from build123d import *

# Parameters (mm, degrees)
F1_DEPTH = 9
F0_R     = 2.5
F2_DEPTH = 2
F3_DEPTH = 6
F4_START = 6
F0_R_2   = 2
F4_DEPTH = 3
F5_W     = 2
F5_H     = 3
F6_DEPTH = 6


with BuildPart() as f1:
    # F0 (on Top) → F1 (new body)
    with BuildSketch(Plane.XY):
        Polygon((-4.9984134711, 16), (-23.5, 16), (-23.5, -16), (-4.9984134711, -16), (4.9998776676, -16), (23.5, -16), (23.5, 16), (4.9998776676, 16), align=None)
        Polygon((-21.5, 11), (-21.5, 14), (-18.5, 14), (18.5, 14), (21.5, 14), (21.5, 11), (21.5, -11), (21.5, -14), (18.5, -14), (-18.5, -14), (-21.5, -14), (-21.5, -11), align=None, mode=Mode.SUBTRACT)
    extrude(amount=F1_DEPTH)

    # F0 (on Top) → F2 (join)
    with BuildSketch(Plane.XY):
        with BuildLine():
            Line((18.5, 14), (-18.5, 14))
            ThreePointArc((-18.5, 14), (-19.3786796564, 11.8786796564), (-21.5, 11))
            Line((-21.5, 11), (-21.5, -11))
            ThreePointArc((-21.5, -11), (-19.3786796564, -11.8786796564), (-18.5, -14))
            Line((-18.5, -14), (18.5, -14))
            ThreePointArc((18.5, -14), (19.3786796564, -11.8786796564), (21.5, -11))
            Line((21.5, -11), (21.5, 11))
            ThreePointArc((21.5, 11), (19.3786796564, 11.8786796564), (18.5, 14))
        make_face()
        with Locations((-11.5, 0)):
            Circle(F0_R, mode=Mode.SUBTRACT)
    extrude(amount=F2_DEPTH)

    # F0 (on Top) → F3 (join)
    with BuildSketch(Plane.XY):
        with BuildLine():
            Line((-18.5, 14), (-21.5, 14))
            Line((-21.5, 14), (-21.5, 11))
            ThreePointArc((-21.5, 11), (-19.3786796564, 11.8786796564), (-18.5, 14))
        make_face()
        with BuildLine():
            Line((21.5, 14), (18.5, 14))
            ThreePointArc((18.5, 14), (19.3786796564, 11.8786796564), (21.5, 11))
            Line((21.5, 11), (21.5, 14))
        make_face()
        with BuildLine():
            Line((21.5, -14), (21.5, -11))
            ThreePointArc((21.5, -11), (19.3786796564, -11.8786796564), (18.5, -14))
            Line((18.5, -14), (21.5, -14))
        make_face()
        with BuildLine():
            ThreePointArc((-18.5, -14), (-19.3786796564, -11.8786796564), (-21.5, -11))
            Line((-21.5, -11), (-21.5, -14))
            Line((-21.5, -14), (-18.5, -14))
        make_face()
    extrude(amount=F3_DEPTH)

    # F0 (on Top) → F4 (join)
    with BuildSketch(Plane.XY.offset(F4_START)):
        with BuildLine():
            Line((-4.9984134711, 20.8740525043), (-4.9984134711, 16))
            Line((-4.9984134711, 16), (4.9998776676, 16))
            Line((4.9998776676, 16), (4.9998776676, 20.9650241638))
            ThreePointArc((4.9998776676, 20.9650241638), (5, 21), (4.9998776676, 21.0349758362))
            ThreePointArc((4.9998776676, 21.0349758362), (-0.0804649964, 25.9993524965), (-4.9984134711, 20.8740525043))
        make_face()
        with Locations((0, 21)):
            Circle(F0_R_2, mode=Mode.SUBTRACT)
        with BuildLine():
            Line((4.9998776676, -16), (-4.9984134711, -16))
            Line((-4.9984134711, -16), (-4.9984134711, -20.8740525043))
            ThreePointArc((-4.9984134711, -20.8740525043), (-0.0804649964, -25.9993524965), (4.9998776676, -21.0349758362))
            Line((4.9998776676, -21.0349758362), (4.9998776676, -20.9650241638))
            Line((4.9998776676, -20.9650241638), (4.9998776676, -16))
        make_face()
        with Locations((0, -21)):
            Circle(F0_R_2, mode=Mode.SUBTRACT)
    extrude(amount=F4_DEPTH)

    # F5 (on face) → F6 (cut)
    with BuildSketch(Plane.XY.offset(9)):
        with Locations((-22.5, 0)):
            Rectangle(F5_W, F5_H)
        with Locations((22.5, 0)):
            Rectangle(F5_W, F5_H)
    extrude(amount=-F6_DEPTH, mode=Mode.SUBTRACT)


solid = f1.part
Read the model definition and answer for the solid it produces. Units are mm, in the model's axes. A direction names the side the tool comes from. Round coordinates to 2 decimals unless told otherwise and drop trailing zeros. Write each loop counter-clockwise with the first axis right and the second up, starting at its lowest first coordinate (ties: lowest second). Pieces come first, ordered by that corner, then holes.
Q1. Find section C-C on z = 0.75. Determine the outline of the cut face in (x, y), and give its area (3 significant figures).
Values:
outline: (-23.5, -16) - (23.5, -16) - (23.5, 16) - (-23.5, 16) - close; hole circle Ø5 at (-11.5, 0)
area: 1,480 mm2
Q2. Find section A-A on y = 0. Determine the outline of the cut face in (x, z).
Values:
outline: (-23.5, 0) - (-14, 0) - (-14, 2) - (-21.5, 2) - (-21.5, 3) - (-23.5, 3) - close; (-9, 0) - (23.5, 0) - (23.5, 3) - (21.5, 3) - (21.5, 2) - (-9, 2) - close
Q3. The mould has two halves that part along X. Classify faces 1 (the face through (-19.4, 11.86, 3.97)), 2 (the face through (0, 0, 0)), 3 (the face through (-23.5, 0, 2)): released by +X, released by -X, zero draft, split by the parting line, or undercut.
Values:
face 1: undercut
face 2: zero draft
face 3: released by -X
Q4. Find section B-B on x = -11.5. Determine the outline of the cut face in (y, z).
Values:
outline: (-16, 0) - (-2.5, 0) - (-2.5, 2) - (-14, 2) - (-14, 9) - (-16, 9) - close; (2.5, 0) - (16, 0) - (16, 9) - (14, 9) - (14, 2) - (2.5, 2) - close
Q5. A tool of negligible diameter and unlimited length cuts with its end or side. For faces 4 (the face through (-0.1, -18.7, 6)), 5 (the face through (-23, 0, 3)), 6 (the face through (20, 13, 6)), 7 (the face through (-4.998, 18, 7)), from which of +Z, -Z, +X, -X, +Y, -Y can it reach the whole face along a straight path? Write none if from no direction.
Values:
face 4: -Z, +X, -X, -Y
face 5: +Z, +X, -X
face 6: +Z
face 7: +Z, -Z, -X, +Y
Q6. Flat-ended cylindrical pins translate along their axes: P1, Ø8, axis at x = 0.5, y = 22.5, coming from the -Z side; P2, Ø1, axis at x = -22, z = 6, coming from the -Y side; P3, Ø3.5, axis at y = -19.5, z = 7, coming from the +X side. Find the tip coordinate at first contact, or state that the pin passes through.
Values:
P1: stops at z = 6
P2: stops at y = -16
P3: stops at x = 5
Q7. Find section D-D on x = 0. Determine the outline of the cut face in (y, z).
Values:
outline: (-26, 6) - (-23, 6) - (-23, 9) - (-26, 9) - close; (-19, 6) - (-16, 6) - (-16, 0) - (16, 0) - (16, 6) - (19, 6) - (19, 9) - (14, 9) - (14, 2) - (-14, 2) - (-14, 9) - (-19, 9) - close; (23, 6) - (26, 6) - (26, 9) - (23, 9) - close
Q8. Straight lines are drawn through the part: line 1 (Y direction, x = -11.5, z = 0.75); line 2 (Y direction, x = 0, z = 8.1); line 3 (Y direction, x = -1.5, z = 5.75). For each, find the intervals that lie inside material, in ascending order.
Values:
line 1: y = -16 to -2.5, 2.5 to 16
line 2: y = -26 to -23, -19 to -14, 14 to 19, 23 to 26
line 3: y = -16 to -14, 14 to 16
